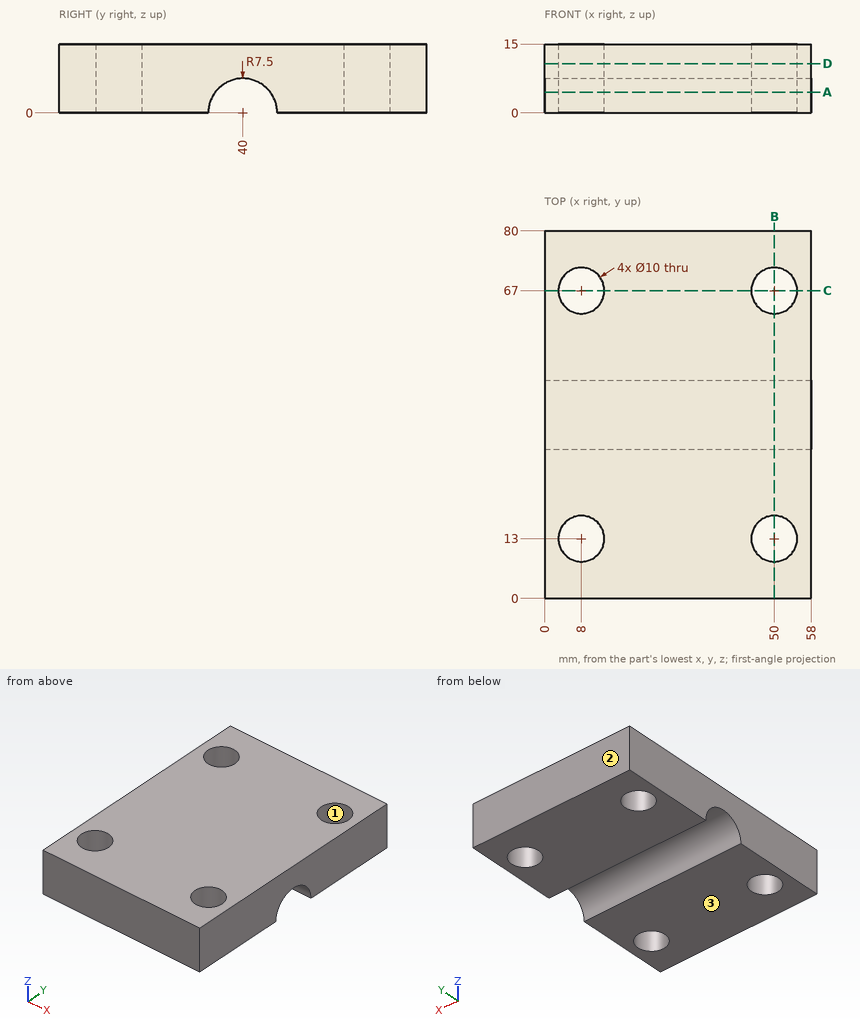
Job drawing, mm, ordinate dimensions from the low corner. One solid piece. Round coordinates to 2 decimals unless told otherwise and drop trailing zeros. Loops run counter-clockwise (first coordinate to the right, second up) from the corner with the lowest first, then second, coordinate; pieces in that order, holes last. Notation, with made-up numbers: (66.5, -27.5) -> (121.5, -27.5) arc R16 cw to (121.5, -11.5) -> close; hole circle Ø7 at (1.5, 37.25). An arc over 180 degrees is marked (long way). Use a Markdown table: item, result.
1) Probe line 1 (Y direction, x = 4, z = 2.25); line 2 (Y direction, x = 9, z = 10); line 3 (Y direction, x = 8, z = 3.5). List the from-to ranges inside material, lowest first. Write a range as [from, to].
The answers:
| item | result |
|---|---|
| line 1 | y = [0, 10], [16, 32.85], [47.15, 64], [70, 80] |
| line 2 | y = [0, 8.1], [17.9, 62.1], [71.9, 80] |
| line 3 | y = [0, 8], [18, 33.37], [46.63, 62], [72, 80] |
2) Pull direction Y, two halves, no side cores. Call the marked faces 1, 2 and 3: pulls with the +Y half, pulls with the -Y half, needs draft (parallel to the pull), parting line crosses it, or undercut.
The answers:
| item | result |
|---|---|
| face 1 | undercut |
| face 2 | pulls with the +Y half |
| face 3 | needs draft |
3) Cut at C-C, the plane y = 67. List the corners of the cut face in (x, z).
The answers:
| item | result |
|---|---|
| outline | (0, 0) -> (3, 0) -> (3, 15) -> (0, 15) -> close; (13, 0) -> (45, 0) -> (45, 15) -> (13, 15) -> close; (55, 0) -> (58, 0) -> (58, 15) -> (55, 15) -> close |
4) Cut at D-D, the plane z = 10.75. List the corners of the cut face in (x, y), and give its area (3 significant figures).
The answers:
| item | result |
|---|---|
| outline | (0, 0) -> (58, 0) -> (58, 80) -> (0, 80) -> close; hole circle Ø10 at (8, 13); hole circle Ø10 at (8, 67); hole circle Ø10 at (50, 13); hole circle Ø10 at (50, 67) |
| area | 4,330 mm2 |
5) Cut at B-B, the plane x = 50. List the corners of the cut face in (y, z).
The answers:
| item | result |
|---|---|
| outline | (0, 0) -> (8, 0) -> (8, 15) -> (0, 15) -> close; (18, 0) -> (32.5, 0) arc R7.5 cw to (47.5, 0) -> (62, 0) -> (62, 15) -> (18, 15) -> close; (72, 0) -> (80, 0) -> (80, 15) -> (72, 15) -> close |
6) Cut at A-A, the plane z = 4.5. List the corners of the cut face in (x, y), and give its area (3 significant figures).
The answers:
| item | result |
|---|---|
| outline | (0, 0) -> (58, 0) -> (58, 34) -> (0, 34) -> close; (0, 46) -> (58, 46) -> (58, 80) -> (0, 80) -> close; hole circle Ø10 at (8, 13); hole circle Ø10 at (8, 67); hole circle Ø10 at (50, 13); hole circle Ø10 at (50, 67) |
| area | 3,630 mm2 |
7) Drop a flat-ended pin along its axis: pin 1 Ø6 at (x, y) = (8, 67) entering from +Z. Give the stop position or say it passes through.
The answers:
| item | result |
|---|---|
| pin 1 | passes through |
